Answer from the drawing. Dimensions are ordinates in mm from the lowest x, y and z of the part. A direction names the side the tool comes from. Give positions to 0.01 mm unless a question says otherwise; leave off trailing zeros. Write each loop counter-clockwise with the first axis right and the second up, starting at its lowest first coordinate (ties: lowest second). Pieces come first, ordered by that corner, then holes. Notation, with made-up numbers: (15.5, 13.5) -> (57.5, 13.5) arc R18 ccw to (57.5, 26.5) -> close; hole circle Ø9 at (9.25, 83). An arc over 180 degrees is marked (long way). Use a Markdown table: item, result. Add a question column.
Q1. Section C-C, the plane y = 1.25 is taken. Give the vertices of the cut face in (x, z), plus the area to 3 significant figures.
Q2. Section B-B, the plane y = 4.5 is taken. Give the vertices of the cut face in (x, z).
Q3. For a pull along X with two mould halves and no side action, classify the marked faces 1, 2, 3 and 4 as pulls with the +X half, pulls with the -X half, needs draft (parallel to the pull), parting line crosses it, or undercut.
Q4. Section A-A, the plane x = 14 is taken. Give the vertices of the cut face in (y, z), plus the area to 3 significant figures.
Q5. Section D-D, the plane z = 24 is taken. Give the vertices of the cut face in (x, y), plus the area to 3 significant figures.
Q6. Each of these flat-tipped pins is pushed along its axis until it touches: pin 1 Ø4 at (x, z) = (14, 14) entering from -Y; pin 2 Ø6 at (x, y) = (14.5, 10.5) entering from -Z; pin 3 Ø5 at (x, z) = (8.5, 10) entering from +Y. Where does it stop, or does it pass through?
Q7. Consider line 1 (X direction, y = 8.25, z = 14); line 2 (Z direction, x = 14, y = 0.8). Determine where each line is inside the solid, lowest interval first.
Q8. For the marked faces 5 and 6, determine the directions among +Z, -Z, +X, -X, +Y, -Y from which every point of the face is accessible in a straight line to the end or side of a thin tool.
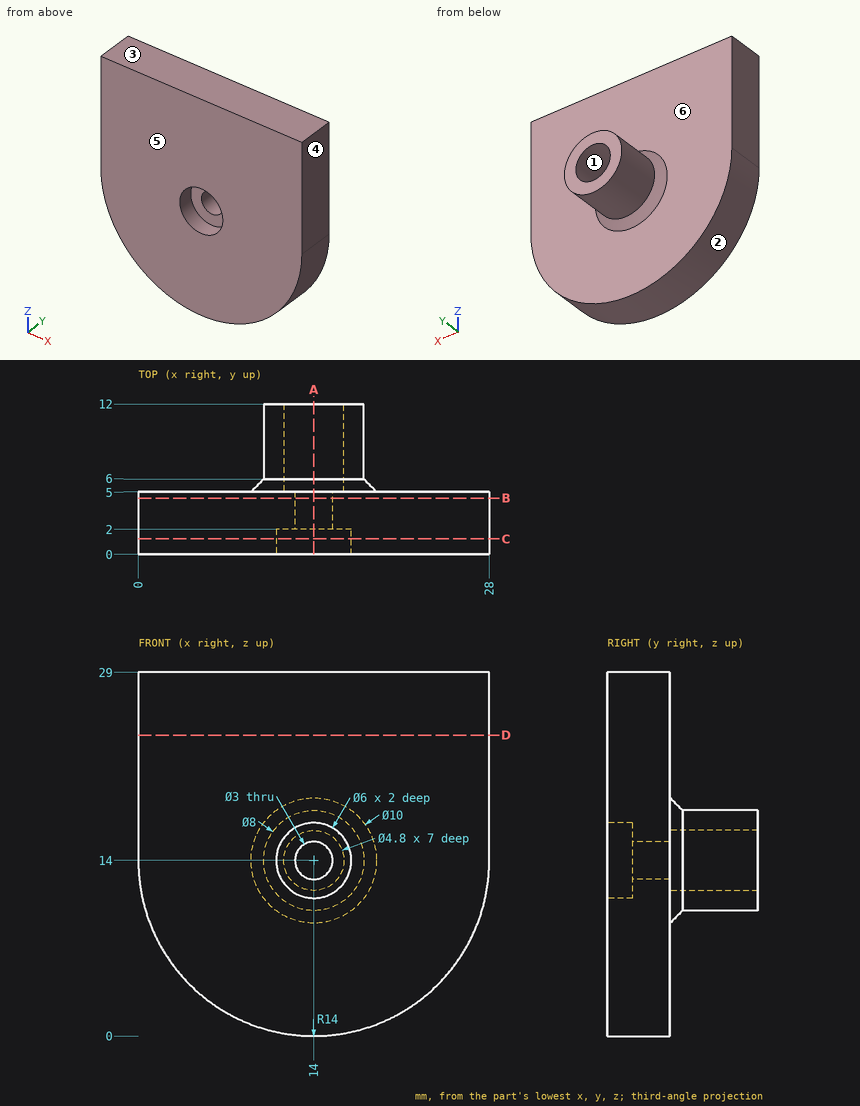
Result set:
| question | item | result |
|---|---|---|
| 1 | outline | (0, 14) arc R14 ccw to (28, 14) -> (28, 29) -> (0, 29) -> close; hole circle Ø6 at (14, 14) |
| 1 | area | 700 mm2 |
| 2 | outline | (0, 14) arc R14 ccw to (28, 14) -> (28, 29) -> (0, 29) -> close; hole circle Ø3 at (14, 14) |
| 3 | face 1 | undercut |
| 3 | face 2 | parting line crosses it |
| 3 | face 3 | needs draft |
| 3 | face 4 | pulls with the +X half |
| 4 | outline | (0, 0) -> (5, 0) -> (5, 9) -> (6, 10) -> (12, 10) -> (12, 11.6) -> (5, 11.6) -> (5, 12.5) -> (2, 12.5) -> (2, 11) -> (0, 11) -> close; (0, 17) -> (2, 17) -> (2, 15.5) -> (5, 15.5) -> (5, 16.4) -> (12, 16.4) -> (12, 18) -> (6, 18) -> (5, 19) -> (5, 29) -> (0, 29) -> close |
| 4 | area | 147 mm2 |
| 5 | outline | (0, 0) -> (28, 0) -> (28, 5) -> (0, 5) -> close |
| 5 | area | 140 mm2 |
| 6 | pin 1 | stops at y = 2 |
| 6 | pin 2 | stops at z = 10 |
| 6 | pin 3 | stops at y = 5.7 |
| 7 | line 1 | x = 10 to 11.6, 16.4 to 18 |
| 7 | line 2 | z = 0 to 11, 17 to 29 |
| 8 | face 5 | +Z, -Z, +X, -X, -Y |
| 8 | face 6 | +Y |
